Autodesk Inventor part; units mm, degrees
ref_plane "Work Plane2" through (-18, -2, 8) normal (0, 0, -1) x (0, 1, 0)
ref_plane "Work Plane3" through (-18, -2, 8) normal (0, 0, -1) x (0, 1, 0)
ref_plane "Work Plane6" through (-18.23, -26.95, 9.05) normal (0, 0, -1) x (0, 1, 0)
ref_plane "Work Plane1" through (0, 0, 0) normal (0, 0, 1) x (1, 0, 0)
sketch "Sketch1" plane through (0, 0, 0) normal (0, 0, 1) x (1, 0, 0)
  circle A0 centre (0, 25) radius 1.95 construction
  circle A1 centre (-25, 0) radius 1.95 construction
  circle A2 centre (-25, -25) radius 1.95 construction
  circle A3 centre (25, 25) radius 1.95 construction
  circle A4 centre (25, -25) radius 1.95 construction
  circle A5 centre (-25, 25) radius 1.95 construction
  circle A6 centre (25, 0) radius 1.95 construction
  circle A7 centre (0, -25) radius 1.95 construction
  line L0 (-28, 30) -> (-30, 28)
  line L1 (-30, 28) -> (-30, -28)
  line L2 (-30, -28) -> (-28, -30)
  line L3 (-28, -30) -> (28, -30)
  line L4 (28, -30) -> (30, -28)
  line L5 (30, -28) -> (30, 28)
  line L6 (30, 28) -> (28, 30)
  line L7 (28, 30) -> (-28, 30)
  circle A8 centre (25, 25) radius 1.45
  circle A9 centre (25, -25) radius 1.45
  circle A10 centre (-25, -25) radius 1.45
  circle A11 centre (-25, 25) radius 1.45
  circle A12 centre (0, 25) radius 1.95
  circle A13 centre (-25, 0) radius 1.95
  circle A14 centre (-25, -25) radius 1.95
  circle A15 centre (25, 25) radius 1.95
  circle A16 centre (25, -25) radius 1.95
  circle A17 centre (-25, 25) radius 1.95
  circle A18 centre (25, 0) radius 1.95
  circle A19 centre (0, -25) radius 1.95
  line L8 (-28, 30) -> (-30, 28)
  line L9 (-30, 28) -> (-30, -28)
  line L10 (-30, -28) -> (-28, -30)
  line L11 (-28, -30) -> (28, -30)
  line L12 (28, -30) -> (30, -28)
  line L13 (30, -28) -> (30, 28)
  line L14 (30, 28) -> (28, 30)
  line L15 (28, 30) -> (-28, 30)
  line L16 (-44.5, 28.8555) -> (-44.5, 2)
  line L17 (-44.5, 34) -> (-45.5, 34)
  line L18 (-45.5, 1) -> (-44.5, 1)
  line L19 (-44.5, 34) -> (-30, 34)
  line L20 (-30, 34) -> (-30, 1)
  line L21 (-30, 1) -> (-44.5, 1)
  line L22 (-44.5, 1) -> (-44.5, 34)
  line L23 (-30, 34) -> (-26, 30)
  line L24 (-30, 34) -> (-24.3431, 34) construction
  point P0 (0, 0)
  dimension "d0" = 2.9
  dimension "d1" = 2.9
  dimension "d2" = 2.9
  dimension "d3" = 2.9
  dimension "d6" = 45
ref_plane "Work Plane2" through (-18, -2, 8) normal (0, 0, -1) x (0, 1, 0)
extrude "Extrusion1" add sketch "Sketch1" along normal blind 3 contours L7 L6 L5 L4 L3 L2 L1 L0 | A12 | A13 | A14 | A15 | A16 | A17 | A18 | A19
sketch "Sketch2" plane through (0, 0, 3) normal (0, 0, 1) x (1, 0, 0)
  arc A0 (7.0684, -7) -> (5.4716, -7) centre (6.27, -5.85) ccw
  arc A1 (5.4716, -21) -> (7.0684, -21) centre (6.27, -22.15) ccw
  line L0 (-18.23, -28.95) -> (30, -28.95)
  line L1 (-18.23, 0.95) -> (30, 0.95)
  line L2 (-18.23, 0.95) -> (30, 0.95)
  line L3 (30, 0.95) -> (30, -28.95)
  line L4 (30, -28.95) -> (-18.23, -28.95)
  line L5 (-18.23, -28.95) -> (-18.23, 0.95)
  circle A2 centre (6.27, -5.85) radius 1.4
  circle A3 centre (6.27, -22.15) radius 1.4
  circle A4 centre (25, -25) radius 1.45
  point P0 (0, 0)
ref_plane "Work Plane3" through (-18, -2, 8) normal (0, 0, -1) x (0, 1, 0)
ref_plane "Work Plane6" through (-18.23, -26.95, 9.05) normal (0, 0, -1) x (0, 1, 0)
extrude "Extrusion2" add sketch "Sketch2" along normal up to surface (6.05 mm away)
sketch "Sketch3" plane through (0, 0, 0) normal (0, 0, -1) x (-1, 0, 0)
  line L0 (-30, -28.95) -> (-30, 0.95)
  line L1 (18.23, -28.95) -> (-30, -28.95)
  line L2 (-30, 0.95) -> (18.23, 0.95)
  line L3 (18.23, 0.95) -> (18.23, -28.95)
  arc A0 (-5.4716, -7) -> (-7.0684, -7) centre (-6.27, -5.85) ccw
  arc A1 (-7.0684, -21) -> (-5.4716, -21) centre (-6.27, -22.15) ccw
  point P0 (0, 0)
hole "Hole2" at (6.27, -22.15, 0) at (6.27, -5.85, 0) direction (0, 0, 1) diameter 3.2 depth 20 tip angle 118 counterbore diameter 5 counterbore depth 4
ref_plane "Work Plane4" through (-44.5, 34, 36.7) normal (0, 1, 0) x (0, 0, -1)
sketch "Sketch5" plane through (-44.5, -30, 36.7) normal (0, 1, 0) x (0, 0, -1)
  line L0 (36.7, -72.5) -> (36.7, -16.5)
  line L1 (36.7, -16.5) -> (33.7, -16.5)
  line L2 (33.7, -72.5) -> (33.7, -16.5)
  line L3 (36.7, -72.5) -> (33.7, -72.5)
  line L4 (25.7, 0) -> (0, 0)
  line L5 (25.7, 0) -> (25.7, 1)
  line L6 (0, 1) -> (25.7, 1)
  line L7 (0, 0) -> (0, 1)
  line L8 (0, 0) -> (24, 0)
  line L9 (24, 0) -> (24, -4)
  line L10 (24, -4) -> (0, -4)
  line L11 (0, -4) -> (0, 0)
  line L12 (24, -4) -> (33.7, -16.5)
  line L13 (36.7, -16.5) -> (36.7, -14.5)
  line L14 (36.7, -14.5) -> (36.7, -16.5)
  line L15 (24, 0) -> (36.7, -14.5)
  line L16 (36.7, -16.5) -> (33.7, -16.5)
  line L17 (36.7, -14.5) -> (36.7, -16.5)
  point P0 (36.7, -44.5)
  dimension "d23" = 24
  dimension "d24" = 4
ref_plane "Work Plane5" through (-45.5, 1, 28.397) normal (0, -1, 0) x (1, 0, 0)
extrude "Extrusion3" add sketch "Sketch5" along normal up to surface (36 mm away) contours L1 L12 L9 L15 L13 | L10 L11 L4 L9
sketch "Sketch6" plane through (-44.5, -30, 36.7) normal (0, -1, 0) x (-1, 0, 0)
  line L0 (-14.5, 36.7) -> (-72.5, 36.7)
  line L1 (-72.5, 36.7) -> (-72.5, 33.7)
  line L2 (-16.5, 33.7) -> (-72.5, 33.7)
  line L3 (-16.5, 33.7) -> (-4, 24)
  line L4 (-4, 24) -> (-4, 0)
  line L5 (-4, 0) -> (0, 0)
  line L6 (0, 0) -> (0, 24)
  line L7 (0, 24) -> (-14.5, 36.7)
  line L8 (-26.27, 27.65) -> (-74.5, 27.65)
  line L9 (-26.27, 33.7) -> (-26.27, 27.65)
  line L10 (-73.55, 33.7) -> (-26.27, 33.7)
  line L11 (-73.55, 33.7) -> (-74.5, 33.7)
  line L12 (-74.5, 33.7) -> (-74.5, 27.65)
  line L13 (-74.5, 27.65) -> (-26.27, 27.65)
  line L14 (-4, 0) -> (-26.27, 27.65)
  line L15 (-26.27, 33.7) -> (-26.27, 27.65)
  line L16 (-26.27, 27.65) -> (-26.27, 33.7)
  line L17 (-26.27, 33.7) -> (-16.5, 33.7)
  line L18 (-16.5, 33.7) -> (-4, 24)
  line L19 (-4, 24) -> (-4, 0)
  point P0 (-44.5, 36.7)
extrude "Extrusion4" add sketch "Sketch6" against normal blind 2 contours L2 L3 L4 L14 L9
sketch "Sketch7" plane through (-44.5, 6, 36.7) normal (-1, 0, 0) x (0, 0, 1)
  circle A0 centre (-2.7, 2.5) radius 1
  circle A1 centre (-7.7, -25.5) radius 1
  circle A2 centre (-23.2, -4) radius 1
  circle A3 centre (-12.7, -15) radius 2.6486
  line L0 (-6.3458, -6.3489) -> (-19.7341, -6.3489)
  line L1 (-19.7341, -6.3489) -> (-19.7341, -23.6095)
  line L2 (-19.7341, -23.6095) -> (-6.3458, -23.6095)
  line L3 (-6.3458, -23.6095) -> (-6.3458, -6.3489)
extrude "Extrusion5" cut sketch "Sketch7" against normal through all contours A0 | A1 | A2 | A3 | L3 L2 L1 L0
sketch "Sketch8" plane through (0, 0, 0) normal (0, 0, -1) x (-1, 0, 0)
  line L0 (-28, 30) -> (28, 30)
  line L1 (-30, 28) -> (-28, 30)
  line L2 (-30, -28) -> (-30, 28)
  line L3 (-28, -30) -> (-30, -28)
  line L4 (30, 28) -> (30, 6)
  line L5 (30, 6) -> (30, -30)
  line L6 (30, -30) -> (-28, -30)
  circle A0 centre (25, -25) radius 1.45
  circle A1 centre (-25, 25) radius 1.45
  circle A2 centre (-25, -25) radius 1.45
  circle A3 centre (25, 25) radius 1.45
  line L7 (71, -30) -> (71, -28)
  line L8 (71, -30) -> (131, 30)
  line L9 (71, -30) -> (155.8528, -30) construction
  line L10 (-28, 30) -> (28, 30)
  line L11 (28, 30) -> (30, 28)
  point P0 (0, 0)
  dimension "d31" = 135
extrude "Extrusion6" [suppressed]
properties part number "cellSTORM_inverted_Laser_left"
The model under review builds one solid part; all positions refer to its coordinate system, in mm. A direction names the side the tool comes from. Round coordinates to 2 decimals unless told otherwise and drop trailing zeros. Loops run counter-clockwise (first coordinate to the right, second up) from the corner with the lowest first, then second, coordinate; pieces in that order, holes last. Notation, with made-up numbers: M 40.25,-1 L 97.25,-1 A14 ccw 97.25,5 Z; hole C 80.25,8.5 d10. An arc over 180 degrees is marked long. Put each result on its own line as item: value.
Q1. Mouldability with a two-part tool opening along Z and no side actions: class faces 5 (the flat face through (6, -28.95, 6)), 6 (the flat face through (-37.35, -12.25, 6.44)), 7 (the flat face through (-43, -0.349, 24)) as released by +Z, released by -Z, zero draft, split by the parting line, or undercut.
Result set:
face 5: zero draft
face 6: released by -Z
face 7: undercut
Q2. Consider section B-B, the plane y = -15. Give the boundary of the cut face in (x, z).
Result set:
outline: M -44.5,12.7 L -30,0 L 30,0 L 30,9.05 L -18.23,9.05 L -18.23,3 L -28,3 L -40.5,12.7 L -40.5,16.97 L -44.5,16.97 Z; M -44.5,30.35 L -40.5,30.35 L -40.5,36.7 L -44.5,36.7 Z
Q3. To check wall thickness, follow L1, parallel to Y at x = -25, z = 2; L2, parallel to Y at x = 6, z = 2; L3, parallel to Z at x = -19, y = 8. State the ranges of each line that lie inside material, in increasing order.
Result set:
L1: y = -30 to -26.45, -23.55 to 23.55, 26.45 to 30
L2: y = -30 to -24.64, -19.66 to -8.34, -3.36 to 30
L3: z = 0 to 3
Q4. Consider section D-D, the plane z = 29. Give the boundary of the cut face in (x, y).
Result set:
outline: M -44.5,-30 L -34.3,-30 L -34.3,-28 L -40.5,-28 L -40.5,-20.5 L -44.5,-20.5 Z; M -44.5,-18.5 L -40.5,-18.5 L -40.5,-17.61 L -44.5,-17.61 Z; M -44.5,-0.35 L -40.5,-0.35 L -40.5,6 L -44.5,6 Z
Q5. For pin 1 (3.5 mm diameter, centred on x = 25, y = -25, fed in from -Z); pin 2 (5 mm diameter, centred on x = 5.5, z = 7, fed in from -Y); pin 3 (1.5 mm diameter, centred on x = -31.5, z = 23.5, fed in from +Y); pin 4 (3 mm diameter, centred on x = 6.27, y = -22.15, fed in from +Z), all flat-tipped, find the tip position at first contact; note any pin that passes through.
Result set:
pin 1: stops at z = 0
pin 2: stops at y = -28.95
pin 3: stops at y = -28
pin 4: passes through
Q6. Consider section C-C, the plane y = 25. Give the boundary of the cut face in (x, z).
Result set:
outline: M -30,0 L -26.45,0 L -26.45,3 L -30,3 Z; M -23.55,0 L 23.55,0 L 23.55,3 L -23.55,3 Z; M 26.45,0 L 30,0 L 30,3 L 26.45,3 Z
Q7. Consider section A-A, the plane x = 6.27. Give the boundary of the cut face in (y, z).
Result set:
outline: M -30,0 L -24.65,0 L -24.65,4 L -23.75,4 L -23.75,9.05 L -28.95,9.05 L -28.95,3 L -30,3 Z; M -20.55,4 L -19.65,4 L -19.65,0 L -8.35,0 L -8.35,4 L -7.45,4 L -7.45,9.05 L -20.55,9.05 Z; M -4.25,4 L -3.35,4 L -3.35,0 L 30,0 L 30,3 L 0.95,3 L 0.95,9.05 L -4.25,9.05 Z
Q8. Machinability: for faces 1 (the flat face through (6, -14, 9.05)), 2 (the flat face through (6, -4, 4)), 3 (the flat face through (-30, 17, 1)), 4 (the flat face through (-43, -9, 30.354)), which of the approach directions +Z, -Z, +X, -X, +Y, -Y give a long, thin tool a straight path to every point of the face, cutting with its end or side? Answer none if there is none.
Result set:
face 1: +Z, +X, +Y, -Y
face 2: -Z
face 3: +Z, -Z, -X, +Y
face 4: +X, -X
